Input: part model. Units: mm. Frame: model coordinates. A direction names the side the tool comes from. Coordinates: 2 decimals unless noted, no trailing zeros. Order: outer loops, then holes, each group sorted by start corner. A loop starts at its lowest first (then second) coordinate and runs counter-clockwise, first axis right, second up. Notation, with made-up numbers: (-28.75, 87) -> (0.25, 87) arc R23 cw to (0.25, 114) -> close; hole circle Ø11 at (88.25, 51). An arc over 180 degrees is marked (long way). One line per question, with ' | ' between items.
```python
from build123d import *

# Parameters (mm, degrees)
SKETCH5_W           = 50.00000000000001
SKETCH5_H           = 130
BOSS_EXTRUDE1_DEPTH = 150
CUT_EXTRUDE1_START  = -25
CUT_EXTRUDE1_DEPTH  = 15
BOSS_EXTRUDE3_START = 30
BOSS_EXTRUDE3_DEPTH = 5
SKETCH10_R          = 8.750000000000018
CUT_EXTRUDE3_DEPTH  = 100
SKETCH18_W          = 48.5
SKETCH18_H          = 10
BOSS_EXTRUDE4_DEPTH = 10
BOSS_EXTRUDE5_START = 40
SKETCH18_2_W        = 48.5
SKETCH18_2_H        = 10
BOSS_EXTRUDE5_DEPTH = 10
CHAMFER1_SIZE       = 25
CUT_EXTRUDE5_DEPTH  = 70
FILLET1_R           = 5
CUT_EXTRUDE6_DEPTH  = 70
FILLET2_R           = 10


with BuildPart() as part:
    # Sketch5 → Boss-Extrude1 (new body)
    with BuildSketch(Plane(origin=(0, 0, 0), x_dir=(1, 0, 0), z_dir=(0, 1, 0))):
        with Locations((25.000000000000004, 65)):
            Rectangle(SKETCH5_W, SKETCH5_H)
    extrude(amount=BOSS_EXTRUDE1_DEPTH)

    # Sketch7 → Cut-Extrude1 (cut, symmetric)
    with BuildSketch(Plane(origin=(50, 0, 0), x_dir=(0, 0, -1), z_dir=(1, 0, 0)).offset(CUT_EXTRUDE1_START)):
        Polygon((130, 0), (130, 133.70233243469318), (0, 42.67535246743131), (0, 0), align=None)
        Polygon((0, 50), (129.99999999999997, 141.02697996726184), (130, 150), (0, 150), align=None)
    extrude(amount=CUT_EXTRUDE1_DEPTH, both=True, mode=Mode.SUBTRACT)

    # Sketch17 → Boss-Extrude3 (add)
    with BuildSketch(Plane(origin=(1.261e-14, 275.41205482615817, -321.9217767956235), x_dir=(1, 0, 0), z_dir=(0, -0.819152044288993, -0.5735764363510444)).offset(BOSS_EXTRUDE3_START)):
        Polygon((9.99999999999999, 374.2932281420449), (39.999999999999986, 374.2932281420449), (39.999999999999986, 334.2932281420449), (9.999999999999993, 334.2932281420449), align=None)
    extrude(amount=-BOSS_EXTRUDE3_DEPTH)

    # Sketch10 → Cut-Extrude3 (cut)
    with BuildSketch(Plane(origin=(0, 33.55050358314182, 23.492315519647676), x_dir=(1, 0, 0), z_dir=(0, 0.819152044288993, 0.5735764363510444))):
        with Locations(Location((25, 68.17827312728308, 0), (0, 0, 90))):
            Circle(SKETCH10_R)
    extrude(amount=-CUT_EXTRUDE3_DEPTH, mode=Mode.SUBTRACT)

    # Sketch18 → Boss-Extrude4 (add)
    with BuildSketch(Plane(origin=(0, 0, 0), x_dir=(0, 0, -1), z_dir=(1, 0, 0))):
        with Locations((24.25, 155)):
            Rectangle(SKETCH18_W, SKETCH18_H)
    extrude(amount=BOSS_EXTRUDE4_DEPTH)

    # Sketch18_2 → Boss-Extrude5 (add)
    with BuildSketch(Plane(origin=(0, 0, 0), x_dir=(0, 0, -1), z_dir=(1, 0, 0)).offset(BOSS_EXTRUDE5_START)):
        with Locations((24.25, 155)):
            Rectangle(SKETCH18_2_W, SKETCH18_2_H)
    extrude(amount=BOSS_EXTRUDE5_DEPTH)

    # Chamfer1
    chamfer1_edges = [part.edges().sort_by_distance(p)[0] for p in [
        (5, 160, 0),
        (45, 160, 0),
    ]]
    chamfer(chamfer1_edges, length=CHAMFER1_SIZE)

    # Sketch21 → Cut-Extrude5 (cut)
    with BuildSketch(Plane(origin=(0, 0, 0), x_dir=(0, 0, -1), z_dir=(1, 0, 0))):
        Polygon((62.424206479876844, 63.19053522493257), (51.526254189207016, 78.75442406642354), (18.76017241764731, 55.81136661238177), (29.65812470831714, 40.2474777708908), align=None)
        Polygon((69.30712371608935, 53.36071069346464), (36.54104194452965, 30.417653239422872), (32.52600689007236, 36.15171754944583), (65.29208866163206, 59.0947750034876), align=None)
    extrude(amount=CUT_EXTRUDE5_DEPTH, mode=Mode.SUBTRACT)

    # Fillet1
    fillet1_edges = [part.edges().sort_by_distance(p)[0] for p in [
        (45, 30.417653239422872, -36.54104194452965),
        (5, 30.417653239422872, -36.54104194452965),
        (45, 40.2474777708908, -29.65812470831714),
        (5.000000000000001, 40.2474777708908, -29.65812470831714),
    ]]
    fillet(fillet1_edges, radius=FILLET1_R)

    # Sketch22 → Cut-Extrude6 (cut)
    with BuildSketch(Plane.ZY):
        Polygon((-115, 0), (-95, 20), (-65, 0), align=None)
    extrude(amount=-CUT_EXTRUDE6_DEPTH, mode=Mode.SUBTRACT)

    # Fillet2
    fillet2_edges = [part.edges().sort_by_distance(p)[0] for p in [
        (25, 50, 0),
    ]]
    fillet(fillet2_edges, radius=FILLET2_R)


solid = part.part
```
1. Ray query, line 1 (X direction, y = 71, z = -87); line 2 (Z direction, x = 5, y = 54); line 3 (Y direction, x = 30.5, z = -39). Return the intervals inside material, ascending. Write a range as [from, to].
Recorded:
line 1: x = [0, 10], [40, 50] | line 2: z = [-130, -68.86], [-58.02, -49.3], [-20.03, 0] | line 3: y = [40.68, 46.79], [75.03, 77.31]
2. Pin query (flat end, axial travel): pin 1 Ø2 at (x, z) = (25, -60) entering from -Y; pin 2 Ø8 at (x, z) = (4.5, -97) entering from +Y; pin 3 Ø3 at (x, y) = (46, 156) entering from -Z. Return the tip coordinate at first contact, or that it passes through.
Recorded:
pin 1: stops at y = 54.69 | pin 2: stops at y = 150 | pin 3: stops at z = -48.5
3. Cut plane A-A, the plane x = 32. Return loops of the section in (y, z).
Recorded:
outline: (36.15, -32.53) -> (45.07, -45.26) -> (49.17, -42.39) -> (40.25, -29.66) -> close; (42.68, 0) -> (64.73, -31.5) -> (69.64, -28.06) -> (52.99, -4.26) arc R10 ccw to (44.79, 0) -> close; (51.09, -53.86) -> (59.09, -65.29) -> (63.19, -62.42) -> (55.19, -51) -> close; (70.75, -40.1) -> (133.7, -130) -> (141.03, -130) -> (75.67, -36.66) -> close
4. Cut plane D-D, the plane y = 118. Return loops of the section in (x, z).
Recorded:
outline: (0, -130) -> (10, -130) -> (10, -107.57) -> (40, -107.57) -> (40, -130) -> (50, -130) -> (50, 0) -> (40, 0) -> (40, -97.11) -> (10, -97.11) -> (10, 0) -> (0, 0) -> close
5. Cut plane C-C, the plane x = 5. Return loops of the section in (y, z), and give its area (3 significant figures).
Recorded:
outline: (0, -130) -> (150, -130) -> (150, -48.5) -> (160, -48.5) -> (160, -25) -> (135, 0) -> (0, 0) -> (0, -65) -> (20, -95) -> (0, -115) -> close; hole (33.29, -40.64) -> (53.36, -69.31) -> (59.09, -65.29) -> (36.15, -32.53) -> (34.51, -33.67) arc R5 ccw to start; hole (43.12, -33.75) -> (63.19, -62.42) -> (78.75, -51.53) -> (55.81, -18.76) -> (44.34, -26.79) arc R5 ccw to start | area: 18,100 mm^2
6. Mould query, pull axis Z, two halves, no side actions, for faces 5 (the face through (41, 67, 0)), 6 (the face through (45, 155, -48.5)), 7 (the face through (4.93, 43.46, -55.17)). Classes: released by +Z, released by -Z, zero draft, split by the parting line, or undercut.
Recorded:
face 5: released by +Z | face 6: released by -Z | face 7: undercut
7. Access query for faces 1 (the face through (45, 10, -105)), 2 (the face through (25.21, 61.11, -63.88)), 3 (the face through (5, 155, -48.5)), 4 (the face through (4.93, 50.158, -22.719)). Directions: +Z, -Z, +X, -X, +Y, -Y. A direction counts if a zero-diameter tool reaches every point of the face in a straight line with its end or side. Return the directions, or none.
Recorded:
face 1: +X, -X, -Y | face 2: -Z | face 3: -Z, +X, -X, +Y | face 4: +X, -X
8. Cut plane B-B, the plane z = -21.5. Return loops of the section in (x, y), and give its area (3 significant figures).
Recorded:
outline: (0, 0) -> (10, 0) -> (10, 51.9) -> (0, 51.9) -> close; (0, 57.73) -> (50, 57.73) -> (50, 156.5) -> (40, 156.5) -> (40, 65.05) -> (10, 65.05) -> (10, 156.5) -> (0, 156.5) -> close; (40, 0) -> (50, 0) -> (50, 51.9) -> (40, 51.9) -> close | area: 3,230 mm^2
